Part model, mm, in its own coordinate system. Face numbers are marked on the shaded views. A direction names the side the tool comes from. Round coordinates to 2 decimals unless told otherwise and drop trailing zeros. Write each loop counter-clockwise with the first axis right and the second up, starting at its lowest first coordinate (ties: lowest second). Pieces come first, ordered by that corner, then holes. Notation, with made-up numbers: M 30.5,-21.75 L 73.5,-21.75 A31 ccw 73.5,11.25 Z; hole C 59.5,60.25 d3. An arc over 180 degrees is marked long. Answer as a JSON object with one key per item and string values. Group by question number.
1. Band-saw the part on C-C, the plane z = 2.25. Write the cut outline in (x, y), plus the area to 3 significant figures.
2. Which spindle directions (+Z, -Z, +X, -X, +Y, -Y) get a long thin tool onto all of the face, cutting with end or side? Do the marked faces 1, 2, 3, 4 and 5. Say none if no direction does.
3. Drill centre lines: line 1 (X direction, y = -95.25, z = 4.2); line 2 (Y direction, x = 19.25, z = 3.85); line 3 (X direction, y = -89, z = 4.75). Where is each one in solid material? Low to high. Write a range as from..to.
4. Band-saw the part on D-D, the plane x = 15. Write the cut outline in (y, z).
5. Drop flat-ended pins along their axis: pin 1 (2 mm diameter, centred on y = -66, z = 1.5, fed in from +X); pin 2 (6 mm diameter, centred on y = -88.5, z = 13.5, fed in from -X); pin 3 (0.9 mm diameter, centred on x = 9.5, z = 1, fed in from -Y). Give the stop position or say it passes through.
6. Two-plate mould, pull along X, no slides. Class the marked faces 6, 7, 8 and 9: +X half, -X half, draft (parallel to the pull), parting line (faces both ways), or undercut.
7. Band-saw the part on A-A, the plane z = 5.75. Write the cut outline in (x, y), plus the area to 3 significant figures.
8. Band-saw the part on B-B, the plane y = -81. Write the cut outline in (x, z), plus the area to 3 significant figures.
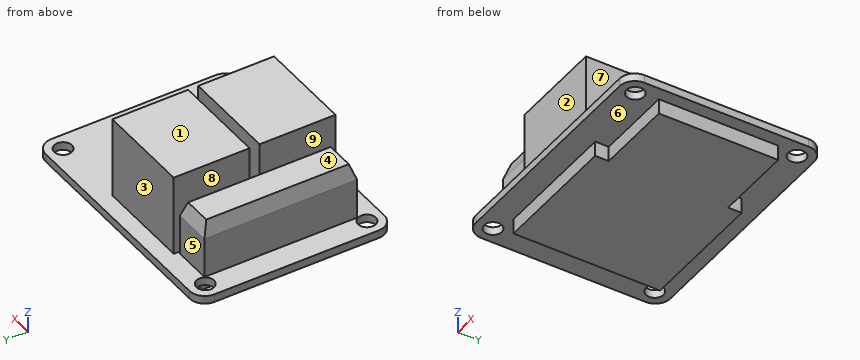
from build123d import *

# Parameters (mm, degrees)
F1_START = 3
F0_W     = 50.5
F0_H     = 38.5
F0_R     = 1.75
F1_DEPTH = 1.6
F2_R     = 3
F3_W     = 15.5
F3_H     = 23.6333997347
F4_DEPTH = 3
F5_W     = 19
F5_H     = 15
F6_DEPTH = 16
F5_W_2   = 7.6
F5_H_2   = 30.2
F7_DEPTH = 11
F8_SIZE2 = 3
F8_SIZE  = 1


with BuildPart() as f1:
    # F0 (on Top) → F1 (new body)
    with BuildSketch(Plane.XY.offset(F1_START)):
        with Locations((-2.75, -79.25)):
            Rectangle(F0_W, F0_H)
        with Locations((-24.75, -95.25)):
            Circle(F0_R, mode=Mode.SUBTRACT)
        with Locations((19.25, -95.25)):
            Circle(F0_R, mode=Mode.SUBTRACT)
        with Locations((-24.75, -63.25)):
            Circle(F0_R, mode=Mode.SUBTRACT)
        with Locations((19.25, -63.25)):
            Circle(F0_R, mode=Mode.SUBTRACT)
    extrude(amount=F1_DEPTH)

    # F2
    f2_edges = [f1.edges().sort_by_distance(p)[0] for p in [
        (22.5, -98.5, 3.8),
        (22.5, -60, 3.8),
        (-28, -60, 3.8),
        (-28, -98.5, 3.8),
    ]]
    fillet(f2_edges, radius=F2_R)

    # F3 (on face) → F4 (join)
    with BuildSketch(Plane(origin=(0, 0, 3), x_dir=(1, 0, 0), z_dir=(0, 0, -1))):
        Polygon((-20.7735065699, 93.75), (-20.7735065699, 64.75), (4.5, 64.75), (4.5, 67.4333001327), (4.5, 91.0666998673), (4.5, 93.75), align=None)
        with Locations((12.25, 79.25)):
            Rectangle(F3_W, F3_H)
    extrude(amount=F4_DEPTH)

    # F5 (on face) → F6 (join)
    with BuildSketch(Plane.XY.offset(4.6)):
        with Locations((-5.5, -70.75)):
            Rectangle(F5_W, F5_H)
        with Locations((-5.5, -87.75)):
            Rectangle(F5_W, F5_H)
    extrude(amount=F6_DEPTH)

    # F5 (on face) → F7 (join)
    with BuildSketch(Plane.XY.offset(4.6)):
        with Locations((-19.3, -79.25)):
            Rectangle(F5_W_2, F5_H_2)
    extrude(amount=F7_DEPTH)

    # F8
    f8_edges = [f1.edges().sort_by_distance(p)[0] for p in [
        (-23.1, -79.25, 15.6),
        (-19.3, -64.15, 15.6),
        (-19.3, -94.35, 15.6),
        (-15.5, -79.25, 15.6),
    ]]
    f8_side = f1.faces().sort_by_distance((-19.3, -79.25, 15.6))[0]
    chamfer(f8_edges, length=F8_SIZE, length2=F8_SIZE2, reference=f8_side)


solid = f1.part
Worked answers:
{
 "1": {"outline": "M -20.77,-93.75 L 4.5,-93.75 L 4.5,-91.07 L 20,-91.07 L 20,-67.43 L 4.5,-67.43 L 4.5,-64.75 L -20.77,-64.75 Z", "area": "1,100 mm^2"},
 "2": {"face 1": "+Z, +X, -X, +Y, -Y", "face 2": "+Z, +X, -X, -Y", "face 3": "+Z, +X, -X, +Y", "face 4": "+Z, -X, +Y, -Y", "face 5": "+Z, -X, +Y"},
 "3": {"line 1": "x = -28..-26.5, -23..17.5, 21..22.5", "line 2": "y = -98.5..-97, -93.5..-65, -61.5..-60", "line 3": "x = -23.1..-15.5, -15..4"},
 "4": {"outline": "M -98.5,3 L -91.07,3 L -91.07,0 L -67.43,0 L -67.43,3 L -60,3 L -60,4.6 L -98.5,4.6 Z"},
 "5": {"pin 1": "stops at x = 4.5", "pin 2": "stops at x = -23.1", "pin 3": "stops at y = -91.07"},
 "6": {"face 6": "draft", "face 7": "+X half", "face 8": "undercut", "face 9": "undercut"},
 "7": {"outline": "M -23.1,-94.35 L -15.5,-94.35 L -15.5,-64.15 L -23.1,-64.15 Z; M -15,-95.25 L 4,-95.25 L 4,-80.25 L -15,-80.25 Z; M -15,-78.25 L 4,-78.25 L 4,-63.25 L -15,-63.25 Z", "area": "800 mm^2"},
 "8": {"outline": "M -28,3 L -20.77,3 L -20.77,0 L 20,0 L 20,3 L 22.5,3 L 22.5,4.6 L 4,4.6 L 4,20.6 L -15,20.6 L -15,4.6 L -15.5,4.6 L -15.5,12.6 L -16.5,15.6 L -22.1,15.6 L -23.1,12.6 L -23.1,4.6 L -28,4.6 Z", "area": "588 mm^2"}
}
